Can you work these out from the model? Positions are in its coordinate system, mm. A direction names the side the tool comes from. Coordinates: 2 decimals unless noted, no trailing zeros. Loops run counter-clockwise (first coordinate to the right, second up) from the corner with the lowest first, then second, coordinate; pieces in that order, holes last. Notation, with made-up numbers: M 53,12.5 L 74,12.5 A30 cw 74,50.5 Z; hole C 48,63.25 d2. An arc over 180 degrees is marked long. Answer as a JSON object with one key per item and string values. Group by question number.
Item 1: Suppose I cut it at D-D (x = -22). Write out the boundary of the cut face in (y, z), then the cut area to 3 significant figures.
Item 2: Suppose I cut it at A-A (z = -11). Write out the boundary of the cut face in (x, y).
Item 3: I'm going to push flat-ended pins straight in: pin 1 Ø1.5 at (y, z) = (6, -3) entering from +X; pin 2 Ø3 at (x, y) = (-26, 8) entering from +Z; pin 3 Ø8 at (x, z) = (32.5, -10) entering from +Y. Where does each tip first touch, or does it pass through?
Item 4: Which directions (+Z, -Z, +X, -X, +Y, -Y) give clear straight access to the entire face, cutting with the end or side of a thin tool? Please do faces 4 (the flat face through (0, 12, -2.4)), 5 (the flat face through (-3, 0, -2)), 6 (the cylindrical face through (-28.57, 0.61, -18.1)), 7 (the flat face through (25.394, 12.325, 0.713)), 8 (the flat face through (19.5, 12, 0)).
Item 5: If I drill on line 1 (X direction, y = 17.25, z = -11.25); line 2 (X direction, y = 6.25, z = -12.75); line 3 (Z direction, x = -34.5, y = 22.75), over which ranges is the centre line in solid material (lowest first)?
Item 6: Suppose I cut it at B-B (x = 18). Write out the boundary of the cut face in (y, z), then the cut area to 4 significant figures.
Item 7: Suppose I cut it at C-C (y = 11.5). Write out the boundary of the cut face in (x, z), then the cut area to 3 significant figures.
Item 8: We'd pull the mould along X, two halves only. Please class faces 1 (the flat face through (23, 12, -19.6)), 2 (the flat face through (3, 25, -2)), 3 (the cylindrical face through (-41, 12, -11)): +X half, -X half, draft (parallel to the pull), parting line (faces both ways), or undercut.
```python
from build123d import *

# Parameters (mm, degrees)
EXTRUDE_THIN1_DEPTH = 25
BOSS_EXTRUDE1_DEPTH = 1.2
BOSS_EXTRUDE2_DEPTH = 25
FILLET1_R           = 1
FILLET2_R           = 5
SKETCH6_W           = 39
SKETCH6_H           = 25
CUT_EXTRUDE1_DEPTH  = 0.5


with BuildPart() as part:
    # Sketch1 → Extrude-Thin1 (new body)
    with BuildSketch(Plane(origin=(0, 0, 0), x_dir=(1, 0, 0), z_dir=(0, 1, 0))):
        with BuildLine():
            Line((0, 0), (-30, 0))
            ThreePointArc((-30, 0), (-41, 11), (-30, 22))
            Line((-30, 22), (-16, 22))
            Line((-16, 22), (-16, 19.6))
            Line((-16, 19.6), (-30, 19.6))
            ThreePointArc((-30, 19.6), (-38.6, 11), (-30, 2.4))
            Line((-30, 2.4), (0, 2.4))
            Line((0, 2.4), (0, 0))
        make_face()
    extrude_thin1 = extrude(amount=EXTRUDE_THIN1_DEPTH)

    # Sketch2 → Boss-Extrude1 (add)
    with BuildSketch(Plane(origin=(0, 0, 0), x_dir=(1, 0, 0), z_dir=(0, 1, 0))):
        with BuildLine():
            Line((-30, 22), (-30, 0))
            ThreePointArc((-30, 0), (-41, 11), (-30, 22))
        make_face()
    boss_extrude1 = extrude(amount=BOSS_EXTRUDE1_DEPTH)

    # Sketch4 → Boss-Extrude2 (add)
    with BuildSketch(Plane(origin=(0, 0, 0), x_dir=(1, 0, 0), z_dir=(0, 1, 0))):
        Polygon((-19.5, 0), (-19.5, -1.5), (-31.456178185, 0.096810325), align=None)
    boss_extrude2 = extrude(amount=BOSS_EXTRUDE2_DEPTH)

    # Mirror1: Extrude-Thin1, Boss-Extrude1, Boss-Extrude2 across plane
    add(extrude_thin1.mirror(Plane(origin=(0, 25, -2.4), x_dir=(0, 0, 1), z_dir=(1, 0, 0))))
    add(boss_extrude1.mirror(Plane(origin=(0, 25, -2.4), x_dir=(0, 0, 1), z_dir=(1, 0, 0))))
    add(boss_extrude2.mirror(Plane(origin=(0, 25, -2.4), x_dir=(0, 0, 1), z_dir=(1, 0, 0))))

    # Fillet1
    fillet1_edges = [part.edges().sort_by_distance(p)[0] for p in [
        (-16, 12.5, -22),
        (-16, 12.5, -19.6),
        (16, 12.5, -19.6),
        (16, 12.5, -22),
    ]]
    fillet(fillet1_edges, radius=FILLET1_R)

    # Fillet2
    fillet2_edges = [part.edges().sort_by_distance(p)[0] for p in [
        (-30, 0.6, -19.6),
        (-30, 0.6, -2.4),
        (30, 0.6, -19.6),
        (30, 0.6, -2.4),
    ]]
    fillet(fillet2_edges, radius=FILLET2_R)

    # Sketch6 → Cut-Extrude1 (cut)
    with BuildSketch(Plane.XY):
        with Locations((0, 12.5)):
            Rectangle(SKETCH6_W, SKETCH6_H)
    extrude(amount=-CUT_EXTRUDE1_DEPTH, mode=Mode.SUBTRACT)


solid = part.part
```
From the geometry:
{
 "1": {"outline": "M 0,-22 L 25,-22 L 25,-19.6 L 0,-19.6 Z; M 0,-2.4 L 25,-2.4 L 25,1.17 L 0,1.17 Z", "area": "149 mm2"},
 "2": {"outline": "M -41,0 L -30,0 L -30,1.2 L -38.6,1.2 L -38.6,25 L -41,25 Z; M 30,0 L 41,0 L 41,25 L 38.6,25 L 38.6,1.2 L 30,1.2 Z"},
 "3": {"pin 1": "x = 38.27", "pin 2": "z = 0.83", "pin 3": "y = 1.2"},
 "4": {"face 4": "+Y", "face 5": "+Z, -Z, +X, -X, -Y", "face 6": "+Y, -Y", "face 7": "+Z, +X, +Y, -Y", "face 8": "+Z, +Y, -Y"},
 "5": {"line 1": "-41 to -38.6, 38.6 to 41", "line 2": "-40.86 to -38.42, 38.42 to 40.86", "line 3": "-21.04 to -18.33, -3.67 to -0.96"},
 "6": {"outline": "M 0,-22 L 25,-22 L 25,-19.6 L 0,-19.6 Z; M 0,-2.4 L 25,-2.4 L 25,-0.5 L 0,-0.5 Z", "area": "107.5 mm2"},
 "7": {"outline": "M -31.46,-0.1 A11 ccw -30,-22 L -17,-22 A1 ccw -16,-21 L -16,-20.6 A1 ccw -17,-19.6 L -30,-19.6 A8.6 cw -30,-2.4 L 30,-2.4 A8.6 cw 30,-19.6 L 17,-19.6 A1 ccw 16,-20.6 L 16,-21 A1 ccw 17,-22 L 30,-22 A11 ccw 31.46,-0.1 L 19.5,1.5 L 19.5,-0.5 L -19.5,-0.5 L -19.5,1.5 Z", "area": "355 mm2"},
 "8": {"face 1": "undercut", "face 2": "draft", "face 3": "-X half"}
}
